from build123d import *

# Parameters (mm, degrees)
SKETCH1_W               = 6
SKETCH1_H               = 6
BOSS_EXTRUDE1_DEPTH     = 4.5
CUT_EXTRUDE1_DEPTH      = 7.184658438
CUT_EXTRUDE1_DEPTH_BACK = 7.184658438
SKETCH2_R               = 1.75
SKETCH3_R               = 1.75
CUT_EXTRUDE2_DEPTH      = 9.077747211
CHAMFER1_SIZE           = 1.5


with BuildPart() as part:
    # Sketch1 → Boss-Extrude1 (new, symmetric)
    with BuildSketch(Plane(origin=(0, 0, 0), x_dir=(1, 0, 0), z_dir=(0, 1, 0))):
        Rectangle(SKETCH1_W, SKETCH1_H)
    extrude(amount=BOSS_EXTRUDE1_DEPTH, both=True)

    # Sketch2 → Cut-Extrude1 (cut, two sides: drawn at the far end of the back side and taken through both)
    with BuildSketch(Plane.XY.offset(-CUT_EXTRUDE1_DEPTH_BACK)):
        with Locations((0, -2)):
            Circle(SKETCH2_R)
    extrude(amount=CUT_EXTRUDE1_DEPTH + CUT_EXTRUDE1_DEPTH_BACK, mode=Mode.SUBTRACT)

    # Sketch3 → Cut-Extrude2 (cut, through all)
    with BuildSketch(Plane.ZY.offset(3)):
        with Locations((0, 2)):
            Circle(SKETCH3_R)
    extrude(amount=-CUT_EXTRUDE2_DEPTH, mode=Mode.SUBTRACT)

    # Chamfer1
    chamfer1_edges = [part.edges().sort_by_distance(p)[0] for p in [
        (0, 4.5, 3),
        (-3, -4.5, 0),
        (3, -4.5, 0),
        (0, 4.5, -3),
    ]]
    chamfer(chamfer1_edges, length=CHAMFER1_SIZE)


solid = part.part
Check sheet for the modelled part. Datum: model origin and axes. Units: mm. Give positions to 0.01 mm unless a question says otherwise; leave off trailing zeros. Write each loop counter-clockwise with the first axis right and the second up, starting at its lowest first coordinate (ties: lowest second). Pieces come first, ordered by that corner, then holes. Notation, with made-up numbers: (3, 27) -> (36, 27) arc R14 cw to (36, 35) -> close; hole circle Ø1 at (36, 79). An arc over 180 degrees is marked (long way). Use one line per item in the form item = value. Start each with the question number.
1. Mould release check, pull along Z, two halves, no side actions. Record for faces 1 (the flat face through (0, 0, 3)), 2 (the flat face through (-2, -4, 0)), 3 (the cylindrical face through (-0.04, 0.29, -0.38)), 4 (the flat face through (0, 4, -2)): pulls with the +Z half, pulls with the -Z half, needs draft (parallel to the pull), parting line crosses it, or undercut.
2. Section check B-B (y = -2). Record the cut outline in (x, z).
3. Section check A-A (x = 0). Record the cut outline in (y, z), and give its area (3 significant figures).
4. Section check D-D (x = 2.75). Record the cut outline in (y, z).
5. Section check C-C (z = 0). Record the cut outline in (x, y).
6. Thickness scan on line 1 along Y through (x, z) = (0, -0.5); line 2 along X through (y, z) = (-2, 1.05); line 3 along Z through (x, y) = (2.5, 3.25). Record the ranges inside material, lowest first. Write a range as from..to.
Conclusion:
q1.face_1 = pulls with the +Z half
q1.face_2 = needs draft
q1.face_3 = undercut
q1.face_4 = pulls with the -Z half
q2.outline = (-3, -3) -> (-1.75, -3) -> (-1.75, 3) -> (-3, 3) -> close; (1.75, -3) -> (3, -3) -> (3, 3) -> (1.75, 3) -> close
q3.outline = (-4.5, -3) -> (-3.75, -3) -> (-3.75, 3) -> (-4.5, 3) -> close; (-0.25, -3) -> (3, -3) -> (4.5, -1.5) -> (4.5, 1.5) -> (3, 3) -> (-0.25, 3) -> close; hole circle Ø3.5 at (2, 0)
q3.area = 21.1 mm²
q4.outline = (-3.25, -3) -> (3, -3) -> (4.5, -1.5) -> (4.5, 1.5) -> (3, 3) -> (-3.25, 3) -> close; hole circle Ø3.5 at (2, 0)
q5.outline = (-3, -3) -> (-1.5, -4.5) -> (1.5, -4.5) -> (3, -3) -> (3, 0.25) -> (-3, 0.25) -> close; (-3, 3.75) -> (3, 3.75) -> (3, 4.5) -> (-3, 4.5) -> close; hole circle Ø3.5 at (0, -2)
q6.line_1 = -4.5..-3.75, -0.25..0.32, 3.68..4.5
q6.line_2 = -3..-1.75, 1.75..3
q6.line_3 = -2.75..-1.22, 1.22..2.75
